Here's how the part is built. I have some questions about the finished solid (model axes, mm). A direction names the side the tool comes from. Give positions to 0.01 mm unless a question says otherwise; leave off trailing zeros. Order: outer loops, then holes, each group sorted by start corner. A loop starts at its lowest first (then second) coordinate and runs counter-clockwise, first axis right, second up. Notation, with made-up numbers: (-34, 2.25) -> (12, 2.25) arc R16 ccw to (12, 7.25) -> close; hole circle Ø5 at (79.5, 49.25). An arc over 180 degrees is marked (long way). Write each question's results on one line, items separated by ' | '. Start each with the question number.
Q1. Imagine slicing it at C-C, the plane x = 1.75. Please give me the cut outline in (y, z) (3 decimals), then the cut area to 3 significant figures.
Q2. For faces 4 (the face through (-0.644, -16.495, -2.166)), 5 (the face through (0.635, -8, 0)), which set-ups out of +Z, -Z, +X, -X, +Y, -Y let a thin tool reach every point of the face, with its end or its side?
Q3. Imagine slicing it at A-A, the plane y = 0. Please give me the cut outline in (x, z) (3 decimals).
Q4. I need wall thicknesses on line 1 along Z through (x, y) = (4.5, 1); line 2 along Y through (x, z) = (9.25, 1.5); line 3 along Z through (x, y) = (2.75, 0.5). Which ranges of each line are inside material? Lowest first, please. Write a range as [from, to].
Q5. Imagine slicing it at B-B, the plane x = 5.5. Please give me the cut outline in (y, z) (3 decimals).
Q6. Thinking about a two-plate mould opening in Y: for faces 1 (the face through (9.906, 3.5, 0.1)), 2 (the face through (-0.331, 9.727, 0.065)), 3 (the face through (3.536, 12.79, -2.84)), which applies, pulls with the +Y half, pulls with the -Y half, needs draft (parallel to the pull), parting line crosses it, or undercut?
Q7. I'm going to push flat-ended pins straight in: pin 1 (3 mm diameter, centred on y = 8, z = 0, fed in from -X); pin 2 (2.5 mm diameter, centred on y = 8.255, z = 0, fed in from -X) (3 decimals); pin 3 (1 mm diameter, centred on x = 3.5, z = 4.5, fed in from -Y); pin 4 (4 mm diameter, centred on y = 0, z = 0, fed in from +X). Where does each tip first touch, or does it pass through?
```python
from build123d import *

# Parameters (mm, degrees)
F3_R     = 3.175
F4_DEPTH = 25.4
F5_R     = 3.81
F7_R     = 1.4732
F8_DEPTH = 1.905


# Not quite as in the source:
# - an extrude whose draft closes it to a point is written as a loft to that point


with BuildPart() as f1:
    # F0 (on Front) → F1 (revolve)
    with BuildSketch(Plane.XZ):
        with BuildLine():
            Line((-1.27, 16.637), (-1.27, 0))
            Line((-1.27, 0), (9.906, 0))
            Line((9.906, 0), (9.906, 5.3514806986))
            ThreePointArc((9.906, 5.3514806986), (9.7616470495, 5.7545817689), (9.3942189832, 5.9744109372))
            ThreePointArc((9.3942189832, 5.9744109372), (5.3425686191, 8.407770264), (3.7717075708, 12.8652924292))
            Line((3.7717075708, 12.8652924292), (0, 16.637))
            Line((0, 16.637), (-1.27, 16.637))
        make_face()
    revolve(axis=Axis((4.318, 0, 0), (1, 0, 0)))

    # F3 (on face) → F4 (cut)
    with BuildSketch(Plane(origin=(-1.27, 0, 0), x_dir=(0, -1, 0), z_dir=(-1, 0, 0))):
        Circle(F3_R)
    extrude(amount=-F4_DEPTH, mode=Mode.SUBTRACT)

    # F5 (on face) → F6 section 0
    with BuildSketch(Plane(origin=(-1.27, 0, 0), x_dir=(0, -1, 0), z_dir=(-1, 0, 0)), mode=Mode.PRIVATE) as f6_s0:
        Circle(F5_R)
    loft([f6_s0.sketch, Vertex(2.54, 0, 0)], ruled=True, mode=Mode.SUBTRACT)

    # F7 (on face) → F8 (cut)
    with BuildSketch(Plane(origin=(-1.27, 0, 0), x_dir=(0, -1, 0), z_dir=(-1, 0, 0))):
        with Locations((-8.255, 0)):
            Circle(F7_R)
        with Locations((8.255, 0)):
            Circle(F7_R)
    extrude(amount=-F8_DEPTH, mode=Mode.SUBTRACT)


solid = f1.part
```
Geometry check:
1) outline: circle Ø29.774 at (0, 0); hole circle Ø6.35 at (0, 0) | area: 665 mm²
2) face 4: +X, -X | face 5: -X
3) outline: (-1.27, -16.637) -> (0, -16.637) -> (3.772, -12.865) arc R6.976 cw to (9.394, -5.974) arc R0.635 ccw to (9.906, -5.351) -> (9.906, -3.175) -> (-0.635, -3.175) -> (-1.27, -3.81) -> close; (-1.27, 3.81) -> (-0.635, 3.175) -> (9.906, 3.175) -> (9.906, 5.351) arc R0.635 ccw to (9.394, 5.974) arc R6.976 cw to (3.772, 12.865) -> (0, 16.637) -> (-1.27, 16.637) -> close
4) line 1: [-9.66, -3.01], [3.01, 9.66] | line 2: [-5.81, -2.8], [2.8, 5.81] | line 3: [-13.88, -3.14], [3.14, 13.88]
5) outline: circle Ø16.443 at (0, 0); hole circle Ø6.35 at (0, 0)
6) face 1: needs draft | face 2: undercut | face 3: parting line crosses it
7) pin 1: x = -1.27 | pin 2: x = 0.635 | pin 3: y = -12.9 | pin 4: through
